Source: CAD feature listing. Evaluate the final solid. Frame: model axes, mm. A direction names the side the tool comes from. Coordinates: 2 decimals unless noted, no trailing zeros. Loops run counter-clockwise (first coordinate to the right, second up) from the corner with the lowest first, then second, coordinate; pieces in that order, holes last.
Item 1: Pin query (flat end, axial travel): pin 1 Ø7.5 at (x, y) = (0, 9.525) entering from +Z (3 decimals); pin 2 Ø1.5 at (x, z) = (-1.5, -4) entering from -Y; pin 3 Ø3 at (x, z) = (0.5, 7) entering from +Y. Return the tip coordinate at first contact, or that it passes through.
Item 2: Pull-direction query (X, two-part tool) for faces 1 (the cylindrical face through (4.44, -23.59, -10.81)), 2 (the flat face through (0, 0, 9.525)), 3 (the cylindrical face through (1.71, 12.2, -10.78)); classes: +X half, -X half, draft (parallel to the pull), parting line (faces both ways), or undercut.
Item 3: Section query A-A, the plane z = -10.25. State how many separate pieces and enclosed holes the cut face has, then the cut area to 3 significant figures.
Item 4: Section query D-D, the plane y = 18. Return the cut outline in (x, z) (3 decimals), then the cut area to 3 significant figures.
Item 5: Reachability of faces 4 (the cylindrical face through (-0.4, 3.02, 0.13)), 5 (the cylindrical face through (-0.688, -12.624, -10.777)) from +Z, -Z, +X, -X, +Y, -Y: full face, straight path, thin tool, end or side. Return the list, or none.
Item 6: Section query C-C, the plane x = -2.5. Return the cut outline in (y, z) (3 decimals), then the cut area to 3 significant figures.
Item 7: Section query B-B, the plane y = 0. Return the cut outline in (x, z) (3 decimals).
Item 8: Line query: probe 1 along Y at (x, z) = (0, -11.35); probe 2 along Z at (x, y) = (-3, 21) (3 decimals); probe 3 along Y at (x, z) = (-0.5, 6.75). Output: solid intervals per line, ascending.
```python
from build123d import *

# Parameters (mm, degrees)
F0_R     = 3.048
F1_DEPTH = 9.525
F2_W     = 12.7
F2_H     = 50.8
F3_DEPTH = 2.54
F4_R     = 6.34999
F5_R     = 1.5875
F5_R_2   = 3.175
F6_DEPTH = 2.541


# Not quite as in the source:
# - a fillet or chamfer is up to 0.001 mm smaller than in the source, because OpenCascade refuses the exact size


with BuildPart() as f1:
    # F0 (on Top) → F1 (new body, symmetric)
    with BuildSketch(Plane.XY):
        Circle(F0_R)
    extrude(amount=F1_DEPTH, both=True)

    # F2 (on face) → F3 (join)
    with BuildSketch(Plane(origin=(0, 0, -9.525), x_dir=(1, 0, 0), z_dir=(0, 0, -1))):
        Rectangle(F2_W, F2_H)
    extrude(amount=F3_DEPTH)

    # F4 (radius 6.35 in the source; OpenCascade refuses exactly that, so slightly less here)
    f4_edges = [f1.edges().sort_by_distance(p)[0] for p in [
        (-6.35, 25.4, -10.795),
        (6.35, 25.4, -10.795),
        (-6.35, -25.4, -10.795),
        (6.35, -25.4, -10.795),
    ]]
    fillet(f4_edges, radius=F4_R)

    # F5 (on face) → F6 (cut, through all)
    with BuildSketch(Plane.XY.offset(-9.525)):
        with Locations((0, 19.05)):
            Circle(F5_R)
        with Locations((0, 9.525)):
            Circle(F5_R_2)
        with Locations((0, -19.05)):
            Circle(F5_R)
        with Locations((0, -9.525)):
            Circle(F5_R_2)
    extrude(amount=-F6_DEPTH, mode=Mode.SUBTRACT)


solid = f1.part
```
Verdict:
1. pin 1: stops at z = -9.525
1. pin 2: stops at y = -2.95
1. pin 3: stops at y = 3.05
2. face 1: +X half
2. face 2: draft
2. face 3: undercut
3. separate pieces: 1
3. enclosed holes: 4
3. area: 531 mm2
4. outline: (-6.35, -12.065) - (-1.191, -12.065) - (-1.191, -9.525) - (-6.35, -9.525) - close; (1.191, -12.065) - (6.35, -12.065) - (6.35, -9.525) - (1.191, -9.525) - close
4. area: 26.2 mm2
5. face 4: +Z
5. face 5: +Z, -Z
6. outline: (-24.887, -12.065) - (-11.482, -12.065) - (-11.482, -9.525) - (-24.887, -9.525) - close; (-7.568, -12.065) - (7.568, -12.065) - (7.568, -9.525) - (1.744, -9.525) - (1.744, 9.525) - (-1.744, 9.525) - (-1.744, -9.525) - (-7.568, -9.525) - close; (11.482, -12.065) - (24.887, -12.065) - (24.887, -9.525) - (11.482, -9.525) - close
6. area: 173 mm2
7. outline: (-6.35, -12.065) - (6.35, -12.065) - (6.35, -9.525) - (3.048, -9.525) - (3.048, 9.525) - (-3.048, 9.525) - (-3.048, -9.525) - (-6.35, -9.525) - close
8. probe 1: y = -25.4 to -20.64, -17.46 to -12.7, -6.35 to 6.35, 12.7 to 17.46, 20.64 to 25.4
8. probe 2: z = -12.065 to -9.525
8. probe 3: y = -3.01 to 3.01
